Autodesk Inventor part; units mm, degrees
ref_plane "YZ Plane" through (0, 0, 0) normal (1, 0, 0) x (0, 1, 0)
ref_plane "XZ Plane" through (0, 0, 0) normal (0, 1, 0) x (-1, 0, 0)
ref_plane "XY Plane" through (0, 0, 0) normal (0, 0, 1) x (1, 0, 0)
sketch "Sketch1" plane through (0, 0, 0) normal (0, 0, 1) x (1, 0, 0)
  line L0 (120.5719, -15.0856) -> (100.5719, -15.0856)
  line L1 (100.5719, -115.0856) -> (120.5719, -115.0856)
  line L2 (125.5719, -110.0856) -> (125.5719, -20.0856)
  line L3 (95.5719, -50.0856) -> (10.5719, -50.0856)
  line L4 (5.5719, -55.0856) -> (5.5719, -75.0856)
  line L5 (10.5719, -80.0856) -> (95.5719, -80.0856)
  line L6 (95.5719, -20.0856) -> (95.5719, -50.0856)
  line L7 (95.5719, -80.0856) -> (95.5719, -110.0856)
  line L8 (125.5719, -65.0856) -> (5.5719, -65.0856) construction
  line L9 (125.5719, -20.0856) -> (120.5719, -15.0856)
  line L10 (100.5719, -15.0856) -> (95.5719, -20.0856)
  line L11 (120.5719, -115.0856) -> (125.5719, -110.0856)
  line L12 (100.5719, -115.0856) -> (95.5719, -110.0856)
  line L13 (10.5719, -80.0856) -> (5.5719, -75.0856)
  line L14 (5.5719, -55.0856) -> (10.5719, -50.0856)
  point P0 (0, 0)
  point P1 (125.5719, -15.0856)
  point P2 (95.5719, -115.0856)
  point P3 (95.5719, -15.0856)
  point P4 (125.5719, -115.0856)
  point P5 (5.5719, -80.0856)
  point P6 (5.5719, -50.0856)
  point P7 (15.5719, -65.0856)
  dimension "d0" = 30
  dimension "d3" = 30
  dimension "d4" = 100
  dimension "d5" = 5
  dimension "d6" = 5
  dimension "d7" = 5
  dimension "d8" = 5
  dimension "d9" = 5
  dimension "d10" = 5
  dimension "d11" = 5
  dimension "d12" = 5
  dimension "d13" = 5
  dimension "d14" = 5
  dimension "d15" = 5
  dimension "d16" = 5
  dimension "d33" = 10
  dimension "d37" = 90
extrude "Extrusion1" add sketch "Sketch1" along normal blind 5
sketch "Sketch2" plane through (0, 0, 5) normal (0, 0, 1) x (1, 0, 0)
  line L0 (5.5719, -55.0856) -> (5.5719, -75.0856)
  line L1 (10.5719, -80.0856) -> (95.5719, -80.0856)
  point P0 (0, 0)
  point P1 (15.5719, -65.0856)
  dimension "d19" = 10
  dimension "d27" = 15
hole "Hole1" at (15.5719, -65.0856, 5) direction (0, 0, -1) diameter 5 end through all
properties part number "PistonV2" material "MDF Medium Density Fiberboard"
The listing builds one solid part. Answer for the finished solid, in the listing's coordinates (mm). A direction names the side the tool comes from. Round coordinates to 2 decimals unless told otherwise and drop trailing zeros. Loops run counter-clockwise (first coordinate to the right, second up) from the corner with the lowest first, then second, coordinate; pieces in that order, holes last.
Q1. Find the intervals of material crossed by line 1 (X direction, y = -30.5, z = 3.55); line 2 (Y direction, x = 51, z = 0.3); line 3 (X direction, y = -78.5, z = 3.65), in increasing order.
Q2. Section A-A, the plane y = -66 is taken. Determine the outline of the cut face in (x, z), then the cut area to 3 significant figures.
Q3. Given pin 1 Ø1 at (x, z) = (28, 2.5) entering from +Y; pin 2 Ø1.5 at (y, z) = (-101, 3.5) entering from -X; pin 3 Ø1.5 at (x, z) = (59, 3.5) entering from -Y, each flat-ended and moving along its own axis, determine where each tip first touches the part or whether it passes through.
Q4. Section B-B, the plane z = 3.9 is taken. Determine the outline of the cut face in (x, y).
Q5. Section D-D, the plane x = 49.5 is taken. Determine the outline of the cut face in (y, z).
Q6. Section C-C, the plane y = -28.5 is taken. Determine the outline of the cut face in (x, z).
Q7. Which of the six approach directions +Z, -Z, +X, -X, +Y, -Y give full straight-line access (tool end or side, diameter ignored) to faces 1 (the face through (54, -50.086, 2)), 2 (the face through (52, -80.086, 2)), 3 (the face through (111, -15.086, 2))?
Completed:
1. line 1: x = 95.57 to 125.57
1. line 2: y = -80.09 to -50.09
1. line 3: x = 8.99 to 125.57
2. outline: (5.57, 0) - (13.25, 0) - (13.25, 5) - (5.57, 5) - close; (17.9, 0) - (125.57, 0) - (125.57, 5) - (17.9, 5) - close
2. area: 577 mm2
3. pin 1: stops at y = -50.09
3. pin 2: stops at x = 95.57
3. pin 3: stops at y = -80.09
4. outline: (5.57, -75.09) - (10.57, -80.09) - (95.57, -80.09) - (95.57, -110.09) - (100.57, -115.09) - (120.57, -115.09) - (125.57, -110.09) - (125.57, -20.09) - (120.57, -15.09) - (100.57, -15.09) - (95.57, -20.09) - (95.57, -50.09) - (10.57, -50.09) - (5.57, -55.09) - close; hole circle Ø5 at (15.57, -65.09)
5. outline: (-80.09, 0) - (-50.09, 0) - (-50.09, 5) - (-80.09, 5) - close
6. outline: (95.57, 0) - (125.57, 0) - (125.57, 5) - (95.57, 5) - close
7. face 1: +Z, -Z, -X, +Y
7. face 2: +Z, -Z, -X, -Y
7. face 3: +Z, -Z, +X, -X, +Y
